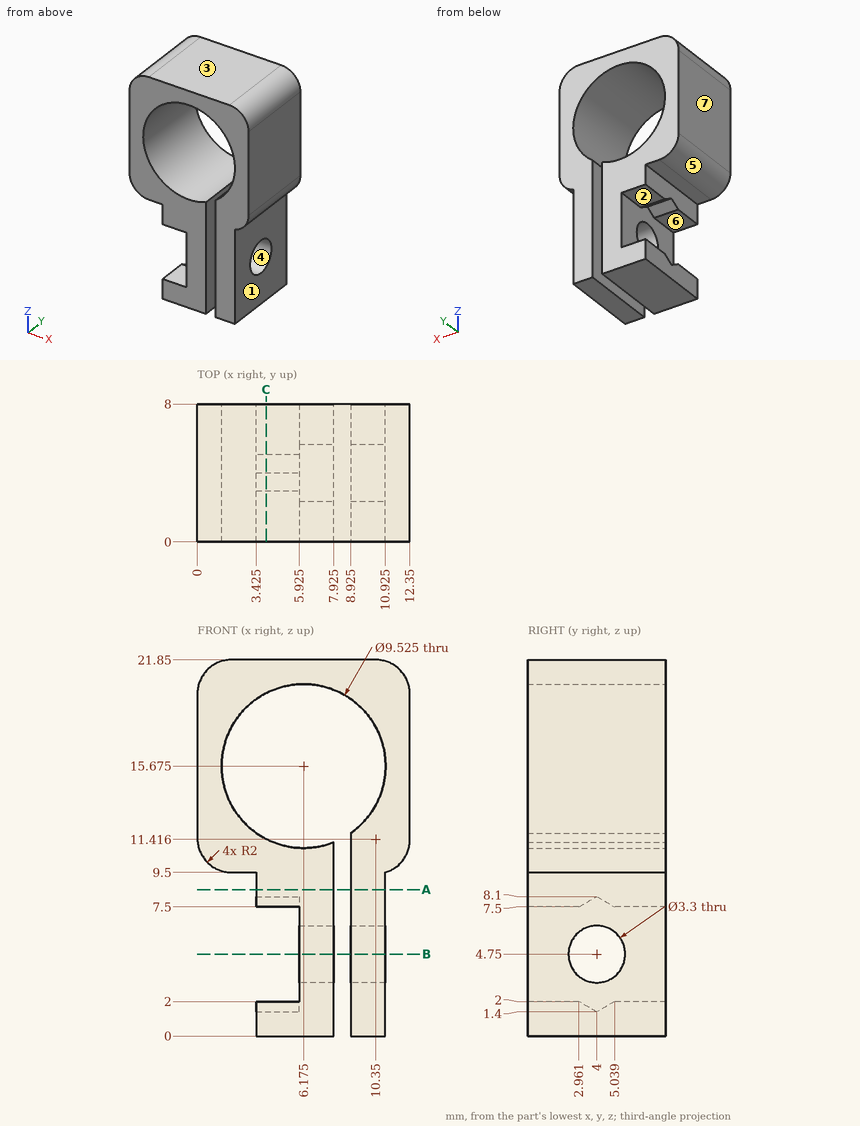
Here's the drawing with two shaded views (mm, measured from the low corner). I have some questions. A direction names the side the tool comes from. Give positions to 0.01 mm unless a question says otherwise; leave off trailing zeros. Order: outer loops, then holes, each group sorted by start corner. A loop starts at its lowest first (then second) coordinate and runs counter-clockwise, first axis right, second up. Notation, with made-up numbers: M 74,-37.75 L 130,-37.75 A31 ccw 130,-3.75 Z; hole C -19,52 d1. An arc over 180 degrees is marked long. Answer as a JSON object with one key per item and string values. Group by question number.
1) Suppose I cut it at C-C, the plane x = 4. Write out the boundary of the cut face in (y, z).
2) I'm going to push flat-ended pins straight in: pin 1 Ø4 at (x, z) = (8.5, 19.5) entering from +Y; pin 2 Ø1.6 at (y, z) = (3.5, 1) entering from -X (3 decimals); pin 3 Ø4 at (y, z) = (4, 4.75) entering from +X (3 decimals); pin 4 Ø1.5 at (y, z) = (7, 3.5) entering from -X (3 decimals). Where does each tip first touch, or does it pass through?
3) We'd pull the mould along Z, two halves only. Please class the marked faces 4, 5, 6 and 7: pulls with the +Z half, pulls with the -Z half, needs draft (parallel to the pull), parting line crosses it, or undercut.
4) On a 3-axis mill with a long thin cutter (end or side, diameter ignored), from which of +Z, -Z, +X, -X, +Y, -Y can I reach the whole of each face in a straight line? I mean the marked faces 1, 2 and 3. Say none if no direction works.
5) Suppose I cut it at B-B, the plane z = 4.75. Count the separate pieces of the cut face and the enclosed holes in it, plus the area to 3 significant figures.
6) Suppose I cut it at A-A, the plane z = 8.5. Write out the boundary of the cut face in (x, y) (1 decimal).
7) Please list where these lines run through material, in increasing order: L1, parallel to X at y = 6.5, z = 8 (1 decimal); L2, parallel to Y at x = 7.5, z = 4.75; L3, parallel to X at y = 0.5, z = 5 (1 decimal). Write a range as [from, to].
Results found:
{
 "1": {"outline": "M 0,0 L 8,0 L 8,2 L 5.04,2 L 4,1.4 L 2.96,2 L 0,2 Z; M 0,7.5 L 2.96,7.5 L 4,8.1 L 5.04,7.5 L 8,7.5 L 8,11.44 L 0,11.44 Z; M 0,19.91 L 8,19.91 L 8,21.85 L 0,21.85 Z"},
 "2": {"pin 1": "y = 8", "pin 2": "x = 3.425", "pin 3": "x = 10.925", "pin 4": "x = 5.925"},
 "3": {"face 4": "undercut", "face 5": "pulls with the -Z half", "face 6": "undercut", "face 7": "needs draft"},
 "4": {"face 1": "-Z, +X, +Y, -Y", "face 2": "-X, +Y, -Y", "face 3": "+Z, +X, -X, +Y, -Y"},
 "5": {"separate pieces": "4", "enclosed holes": "0", "area": "18.8 mm²"},
 "6": {"outline": "M 3.4,0 L 7.9,0 L 7.9,8 L 3.4,8 Z; M 8.9,0 L 10.9,0 L 10.9,8 L 8.9,8 Z"},
 "7": {"L1": "[3.4, 7.9], [8.9, 10.9]", "L2": "[0, 2.35], [5.65, 8]", "L3": "[5.9, 7.9], [8.9, 10.9]"}
}
